Autodesk Inventor part; units mm, degrees
ref_plane "Work Plane1" through (0, 0, -15) normal (0, 0, 1) x (1, 0, 0)
ref_plane "YZ Plane" through (0, 0, 0) normal (1, 0, 0) x (0, 1, 0)
ref_plane "XZ Plane" through (0, 0, 0) normal (0, 1, 0) x (-1, 0, 0)
sketch "Sketch1" plane through (0, 0, 0) normal (0, 0, 1) x (1, 0, 0)
  line L0 (0, 0) -> (25, 0)
  line L1 (25, 0) -> (25, 40)
  line L2 (25, 40) -> (0, 40)
  line L3 (0, 40) -> (0, 0)
  dimension "d1" = 25
  dimension "d2" = 40
  dimension "d3" = 25
extrude "Extrusion1" add sketch "Sketch1" against normal blind 30
sketch "Sketch2" plane through (25, 0, 0) normal (1, 0, 0) x (0, 0, -1)
  line L0 (0, 0) -> (30, 0)
  circle A0 centre (15, 6.56) radius 2.46
extrude "Extrusion2" cut sketch "Sketch2" against normal blind 30
sketch "Sketch3" plane through (0, 0, 0) normal (-1, 0, 0) x (0, 0, 1)
  line L0 (0, 0) -> (-30, 0)
  line L1 (-25.05, 0) -> (-4.95, 0)
  line L2 (-4.95, 0) -> (-4.95, 33.12)
  line L3 (-4.95, 33.12) -> (-25.05, 33.12)
  line L4 (-25.05, 33.12) -> (-25.05, 0)
  dimension "d11" = 20.1
extrude "Extrusion3" cut sketch "Sketch3" against normal blind 20
sketch "Sketch4" plane through (0, 0, 0) normal (0, -1, 0) x (1, 0, 0)
  line L0 (20, -4.95) -> (20, -25.05)
  line L1 (20, -15) -> (25, -15)
  line L2 (25, 0) -> (25, -30)
  line L3 (20, -8.025) -> (25, -8.025)
  line L4 (25, -8.025) -> (25, -21.975)
  line L5 (25, -21.975) -> (20, -21.975)
  line L6 (20, -21.975) -> (20, -8.025)
  line L7 (20, -8.025) -> (25, -21.975) construction
  line L8 (25, -8.025) -> (20, -21.975) construction
  line L9 (25, -12.54) -> (25, -17.46)
  point P0 (0, 0)
  point P1 (22.5, -15)
  dimension "d14" = 13.95
extrude "Extrusion4" add sketch "Sketch4" along normal blind 15
sketch "Sketch5" plane through (20, 0, 0) normal (-1, 0, 0) x (0, 0, 1)
  circle A0 centre (-15, 6.56) radius 2.46
  circle A1 centre (-15, 6.56) radius 4.7025
  circle A2 centre (-15, 6.56) radius 2.46
  circle A3 centre (-15, 6.56) radius 2.46
  point P0 (0, 0)
  dimension "d17" = 9.405
extrude "Extrusion5" cut sketch "Sketch5" against normal blind 2.1
sketch "Sketch6" plane through (25, 0, 0) normal (1, 0, 0) x (0, 0, -1)
  circle A0 centre (15, 6.56) radius 4.7025
  line L0 (15, 6.56) -> (15, 23.56)
  circle A1 centre (15, 23.56) radius 2.46
  point P0 (0, 0)
  dimension "d20" = 17
  dimension "d21" = 4.92
extrude "Extrusion6" cut sketch "Sketch6" against normal blind 10 contours A1
sketch "Sketch7" plane through (20, 0, 0) normal (-1, 0, 0) x (0, 0, 1)
  circle A0 centre (-15, 23.56) radius 2.46
  circle A1 centre (-15, 23.56) radius 4.7025
  point P0 (0, 0)
  dimension "d24" = 9.405
extrude "Extrusion7" cut sketch "Sketch7" against normal blind 2.1
sketch "Sketch9" plane through (25, 0, 0) normal (1, 0, 0) x (0, 0, -1)
  circle A0 centre (15, 6.56) radius 2.46
  circle A1 centre (15, 6.56) radius 2.46
  circle A2 centre (15, 23.56) radius 2.46
  circle A3 centre (15, 23.56) radius 2.46
  line L0 (30, 40) -> (30, 0)
  line L1 (30, 0) -> (30, 40)
  line L2 (30, 40) -> (0, 40)
  line L3 (0, 40) -> (0, 0)
  line L4 (0, 0) -> (8.025, 0)
  line L5 (21.975, 0) -> (21.975, -15)
  line L6 (21.975, -15) -> (8.025, -15)
  line L7 (8.025, -15) -> (8.025, 0)
  line L8 (0, 0) -> (8.025, 0)
  line L9 (21.975, 0) -> (30, 0)
extrude "Extrusion8" add sketch "Sketch9" along normal blind 5
sketch "Sketch10" plane through (0, 40, 0) normal (0, 1, 0) x (1, 0, 0)
  line L0 (0, 30) -> (30, 30)
  line L1 (30, 0) -> (0, 0)
  line L2 (0, 30) -> (30, 30)
  line L3 (30, 30) -> (30, 0)
  line L4 (30, 0) -> (0, 0)
  line L5 (0, 0) -> (0, 30)
extrude "Extrusion9" add sketch "Sketch10" along normal blind 30
sketch "Sketch12" plane through (30, 0, 0) normal (1, 0, 0) x (0, 0, -1)
  circle A0 centre (15, 6.56) radius 2.46
  line L0 (15, 6.56) -> (15, 15.06)
  circle A1 centre (15, 15.06) radius 2.525
  point P0 (0, 0)
  dimension "d31" = 8.5
  dimension "d33" = 5.05
extrude "Extrusion10" cut sketch "Sketch12" against normal blind 30 contours A1
sketch "Sketch14" plane through (0, 0, 0) normal (0, 0, 1) x (1, 0, 0)
  line L0 (30, 70) -> (0, 70)
  line L1 (0, 70) -> (0, 85)
  line L2 (-15, 100) -> (-23, 100)
  line L3 (30, 0) -> (30, 70)
  line L4 (30, 122.5) -> (30, 70)
  arc A0 (0, 85) -> (-15, 100) centre (-15, 85) ccw
  line L5 (30, 105) -> (30, 100)
  line L6 (-23, 145) -> (15, 145)
  line L7 (-18, 142.5) -> (-23, 145)
  line L8 (-18, 102.5) -> (-23, 100)
  line L9 (-18, 102.5) -> (-13, 122.5)
  line L10 (-13, 122.5) -> (-18, 142.5)
  line L11 (30, 122.5) -> (15, 145)
  point P0 (0, 0)
  point P1 (0, 100)
  dimension "d47" = 30
  dimension "d54" = 15
extrude "Extrusion12" add sketch "Sketch14" against normal blind 30
sketch "Sketch15" plane through (0, 0, -25.05) normal (-1, 0, 0) x (0, 0, 1)
  line L0 (0, 33.12) -> (20.1, 33.12)
  line L1 (20.1, 33.12) -> (20.1, 0)
  line L2 (0, 33.12) -> (20.1, 33.12)
  line L3 (20.1, 33.12) -> (20.1, 31.1)
  line L4 (20.1, 31.1) -> (0, 31.1)
  line L5 (0, 31.1) -> (0, 33.12)
  point P0 (25.05, 0)
  dimension "d57" = 2.02
extrude "Extrusion13" add sketch "Sketch15" against normal blind 20
sketch "Sketch24" plane through (0, 0, 0) normal (0, 0, 1) x (1, 0, 0)
  line L0 (-15, 100) -> (-23, 100)
  line L1 (-15, 100) -> (-23, 100)
  line L2 (-23, 100) -> (-18, 102.5)
  line L3 (-23, 100) -> (-18, 102.5)
  line L4 (-18, 102.5) -> (-13, 122.5)
  line L5 (-18, 102.5) -> (-13, 122.5)
  line L6 (-13, 122.5) -> (-18, 142.5)
  line L7 (-13, 122.5) -> (-18, 142.5)
  line L8 (-18, 142.5) -> (-23, 145)
  line L9 (-18, 142.5) -> (-23, 145)
  line L10 (-23, 145) -> (15, 145)
  line L11 (-23, 145) -> (15, 145)
  line L12 (15, 145) -> (30, 122.5)
  line L13 (15, 145) -> (30, 122.5)
  line L14 (30, 122.5) -> (30, 77.5)
  line L15 (30, 0) -> (30, 122.5)
  line L16 (30, 77.5) -> (0, 77.5)
  line L17 (0, 0) -> (0, 85)
  line L18 (0, 77.5) -> (0, 85)
  arc A0 (0, 85) -> (-15, 100) centre (-15, 85) ccw
  arc A1 (0, 85) -> (-15, 100) centre (-15, 85) ccw
  dimension "d86" = 45
extrude "Extrusion14" add sketch "Sketch24" along normal blind 30
ref_plane "Work Plane1" through (0, 0, -15) normal (0, 0, 1) x (1, 0, 0)
mirror "Mirror1" about plane through (0, 0, -15) normal (0, 0, 1) of "Extrusion14"
properties part number "rec_a_40mm_x_90mm"
Can you work these out from the model? Positions are in its coordinate system, mm. A direction names the side the tool comes from. Coordinates: 2 decimals unless noted, no trailing zeros. Write each loop counter-clockwise with the first axis right and the second up, starting at its lowest first coordinate (ties: lowest second). Pieces come first, ordered by that corner, then holes. Notation, with made-up numbers: (13, 24.25) - (44, 24.25) arc R7 ccw to (44, 29.25) - close; hole circle Ø10 at (71, 54.25). An arc over 180 degrees is marked (long way). Return JSON: item names as keys, results as strings. Group by question number.
Item 1: Which directions (+Z, -Z, +X, -X, +Y, -Y) give clear straight access to the entire face, cutting with the end or side of a thin tool? Please do faces 1 (the face through (15, 77.5, -45)), 2 (the face through (-15.465, 112.64, -14.37)), 3 (the face through (10, 31.1, -15)), 4 (the face through (25, -8, -8.025)).
Item 2: I'm going to push flat-ended pins straight in: pin 1 Ø22 at (x, y) = (9.5, 8) entering from +Z; pin 2 Ø4.5 at (y, z) = (5, -17) entering from -X; pin 3 Ø9 at (x, z) = (17.5, 19) entering from -Y. Where does each tip first touch, or does it pass through?
Item 3: If we section it at B-B (z = -15.5): Count the separate pieces of the cut face and the enclosed holes in it, then the cut area to 3 significant figures.
Item 4: If we section it at A-A (y = 6.56): Write out the boundary of the cut face in (x, z).
Item 5: If we section it at C-C (x = 5.5): Write out the boundary of the cut face in (y, z), then the cut area to 3 significant figures.
Item 6: If we section it at D-D (z = 6): Write out the boundary of the cut face in (x, y).
Item 7: We'd pull the mould along Z, two halves only. Please class faces 5 (the face through (25, -7, -21.975)), 6 (the face through (10, 15, -4.95)), 7 (the face through (21.035, 27.525, -12.472)), 8 (the face through (18, 0, -27)): pulls with the +Z half, pulls with the -Z half, needs draft (parallel to the pull), parting line crosses it, or undercut.
Item 8: Please list where these lines run through material, in increasing order: probe 1 along Z at (x, y) = (26.75, 6.56); probe 2 along Z at (x, y) = (8.5, 5); probe 3 along Y at (x, z) = (26.5, -15) (3 decimals).
Return value:
{
 "1": {"face 1": "-Z, +X, -X, -Y", "face 2": "+Z, -Z, -X", "face 3": "-X, -Y", "face 4": "+Z, +X, -X, -Y"},
 "2": {"pin 1": "stops at z = 0", "pin 2": "stops at x = 20", "pin 3": "stops at y = 77.5"},
 "3": {"separate pieces": "4", "enclosed holes": "0", "area": "4,320 mm^2"},
 "4": {"outline": "(0, -30) - (30, -30) - (30, -17.46) - (22.1, -17.46) - (22.1, -19.7) - (20, -19.7) - (20, -25.05) - (0, -25.05) - close; (0, -4.95) - (20, -4.95) - (20, -10.3) - (22.1, -10.3) - (22.1, -12.54) - (30, -12.54) - (30, 0) - (0, 0) - close"},
 "5": {"outline": "(0, -30) - (77.5, -30) - (77.5, -60) - (145, -60) - (145, 30) - (77.5, 30) - (77.5, 0) - (0, 0) - (0, -4.95) - (31.1, -4.95) - (31.1, -25.05) - (0, -25.05) - close", "area": "7,770 mm^2"},
 "6": {"outline": "(-23, 100) - (-15, 100) arc R15 cw to (0, 85) - (0, 77.5) - (30, 77.5) - (30, 122.5) - (15, 145) - (-23, 145) - (-18, 142.5) - (-13, 122.5) - (-18, 102.5) - close"},
 "7": {"face 5": "pulls with the -Z half", "face 6": "undercut", "face 7": "undercut", "face 8": "needs draft"},
 "8": {"probe 1": "z = -30 to -17.46, -12.54 to 0", "probe 2": "z = -30 to -25.05, -4.95 to 0", "probe 3": "y = -15 to 4.1, 9.02 to 12.535, 17.585 to 21.1, 26.02 to 127.75"}
}
